Check sheet for the modelled part. Datum: model origin and axes. Units: mm. A direction names the side the tool comes from. Give positions to 0.01 mm unless a question says otherwise; leave off trailing zeros. Loops run counter-clockwise (first coordinate to the right, second up) from the corner with the lowest first, then second, coordinate; pieces in that order, holes last. Notation, with made-up numbers: (-10.5, -5) - (-5.5, -5) arc R15 ccw to (-5.5, 9) - close; hole circle Ø6 at (31, 18.5). An arc over 180 degrees is marked (long way). Use one line per item in the form item = value.
from build123d import *

# Parameters (mm, degrees)
BOSS_EXTRUDE1_DEPTH     = 8.5
CUT_EXTRUDE1_DEPTH      = 2
CUT_EXTRUDE1_DEPTH_BACK = 26.602245995
SKETCH2_R               = 2.75
CUT_EXTRUDE2_DEPTH      = 2
CUT_EXTRUDE2_DEPTH_BACK = 0.25
SKETCH2_3_R             = 5
SKETCH2_3_R_2           = 2.75
SKETCH3_R               = 1.75
CUT_EXTRUDE3_DEPTH      = 28.391148205
SKETCH3_3_R             = 3
SKETCH3_3_R_2           = 1.75
CUT_EXTRUDE4_DEPTH      = 5.85
FILLET1_R               = 2
FILLET2_R               = 2
CUT_EXTRUDE5_DEPTH      = 2
SKETCH5_R               = 1.2
BOSS_EXTRUDE2_DEPTH     = 4
FILLET3_R               = 1
FILLET4_R               = 0.5


with BuildPart() as part:
    # Sketch1 → Boss-Extrude1 (new, symmetric)
    with BuildSketch(Plane.XY):
        with BuildLine():
            Line((11.05, 4), (3.970201506, 4))
            ThreePointArc((3.970201506, 4), (-3.590264914, 6.674165907), (2.926174978, 2))
            Line((2.926174978, 2), (22.05, 2))
            Line((22.05, 2), (22.05, -2))
            Line((22.05, -2), (-22.05, -2))
            Line((-22.05, -2), (-22.05, 2))
            Line((-22.05, 2), (-9.85, 2))
            ThreePointArc((-9.85, 2), (-7.870101013, 2.820101013), (-7.05, 4.8))
            ThreePointArc((-7.05, 4.8), (-1.645444408, 11.655290855), (6.281918497, 8))
            Line((6.281918497, 8), (11.05, 8))
            Line((11.05, 8), (11.05, 4))
        make_face()
    extrude(amount=BOSS_EXTRUDE1_DEPTH, both=True)

    # Sketch2 → Cut-Extrude1 (cut, two sides: drawn at the far end of the back side and taken through both)
    with BuildSketch(Plane(origin=(0, 2, 0), x_dir=(1, 0, 0), z_dir=(0, 1, 0)).offset(-CUT_EXTRUDE1_DEPTH_BACK)):
        with Locations(Location((16.3, 0, 0), (0, 0, 180))):
            Circle(SKETCH2_R)
        with Locations(Location((-16.3, 0, 0), (0, 0, 180))):
            Circle(SKETCH2_R)
    extrude(amount=CUT_EXTRUDE1_DEPTH + CUT_EXTRUDE1_DEPTH_BACK, mode=Mode.SUBTRACT)

    # Sketch2<3> → Cut-Extrude2 (cut, two sides: drawn at the far end of the back side and taken through both)
    # profile 1 of 2: a face of its own
    with BuildSketch(Plane(origin=(0, 2, 0), x_dir=(1, 0, 0), z_dir=(0, 1, 0)).offset(-CUT_EXTRUDE2_DEPTH_BACK)):
        with Locations(Location((16.3, 0, 0), (0, 0, 180))):
            Circle(SKETCH2_3_R)
        with Locations(Location((16.3, 0, 0), (0, 0, 180))):
            Circle(SKETCH2_3_R_2, mode=Mode.SUBTRACT)
    # profile 2 of 2: a face of its own
    with BuildSketch(Plane(origin=(0, 2, 0), x_dir=(1, 0, 0), z_dir=(0, 1, 0)).offset(-CUT_EXTRUDE2_DEPTH_BACK)):
        with Locations(Location((-16.3, 0, 0), (0, 0, 180))):
            Circle(SKETCH2_3_R)
        with Locations(Location((-16.3, 0, 0), (0, 0, 180))):
            Circle(SKETCH2_3_R_2, mode=Mode.SUBTRACT)
    extrude(amount=CUT_EXTRUDE2_DEPTH + CUT_EXTRUDE2_DEPTH_BACK, mode=Mode.SUBTRACT)

    # Sketch3 → Cut-Extrude3 (cut, through all)
    with BuildSketch(Plane(origin=(0, 11.85, 0), x_dir=(1, 0, 0), z_dir=(0, 1, 0))):
        with Locations(Location((7.510100753, 0, 0), (0, 0, 225.426920251))):
            Circle(SKETCH3_R)
    extrude(amount=-CUT_EXTRUDE3_DEPTH, mode=Mode.SUBTRACT)

    # Sketch3<3> → Cut-Extrude4 (cut)
    # profile 1 of 2: a face of its own
    with BuildSketch(Plane(origin=(0, 11.85, 0), x_dir=(1, 0, 0), z_dir=(0, 1, 0))):
        with Locations(Location((7.510100753, 0, 0), (0, 0, 245.83322212))):
            Circle(SKETCH3_3_R)
        with Locations(Location((7.510100753, 0, 0), (0, 0, 180))):
            Circle(SKETCH3_3_R_2, mode=Mode.SUBTRACT)
    # profile 2 of 2: a face of its own
    with BuildSketch(Plane(origin=(0, 11.85, 0), x_dir=(1, 0, 0), z_dir=(0, 1, 0))):
        with Locations(Location((7.510100753, 0, 0), (0, 0, 180))):
            Circle(SKETCH3_3_R_2)
    extrude(amount=-CUT_EXTRUDE4_DEPTH, mode=Mode.SUBTRACT)

    # Fillet1
    fillet1_edges = [part.edges().sort_by_distance(p)[0] for p in [
        (22.05, 0, 8.5),
        (-22.05, 0, -8.5),
        (-22.05, 0, 8.5),
    ]]
    fillet(fillet1_edges, radius=FILLET1_R)

    # Fillet2
    # the kernel refuses this fillet: 2 mm, written as the material it adds along each edge
    with BuildSketch(Plane(origin=(6.281918497, 8, -0.075436901), x_dir=(1, 0, 0), z_dir=(0, 0, 1))) as fillet2_piece_1_section:
        with BuildLine():
            CenterArc((1.125003941, 2), FILLET2_R, 215.07061915, 54.92938085)
            ThreePointArc((-0.511884995, 0.850828729), (-0.240944724, 0.434437491), (0, 0))
            Line((0, 0), (1.125003941, 0))
        make_face()
    fillet2_piece_1 = extrude(amount=8.575436901, mode=Mode.PRIVATE)
    fillet2_piece_1 = fillet2_piece_1 - Plane(origin=(7.510100753, 8.184515376, 0), x_dir=(-0.4093940854484991, 0, 0.9123576507049125), z_dir=(0, 1, 0)) * Cylinder(3, 22, mode=Mode.PRIVATE)
    add(fillet2_piece_1)
    with BuildSketch(Plane(origin=(6.281918497, 8, -8.5), x_dir=(1, 0, 0), z_dir=(0, 0, 1))) as fillet2_piece_2_section:
        with BuildLine():
            CenterArc((1.125003941, 2), FILLET2_R, 215.07061915, 54.92938085)
            ThreePointArc((-0.511884995, 0.850828729), (-0.240944724, 0.434437491), (0, 0))
            Line((0, 0), (1.125003941, 0))
        make_face()
    fillet2_piece_2 = extrude(amount=8.575436901, mode=Mode.PRIVATE)
    fillet2_piece_2 = fillet2_piece_2 - Plane(origin=(7.510100753, 8.184515325, 0), x_dir=(-0.4093940854484991, 0, 0.9123576507049125), z_dir=(0, 1, 0)) * Cylinder(3, 22, mode=Mode.PRIVATE)
    add(fillet2_piece_2)
    # the kernel refuses this fillet: 2 mm, written as the material it takes off along each edge
    with BuildSketch(Plane(origin=(11.05, 13, -8.5), x_dir=(-1, 0, 0), z_dir=(0, -1, 0))) as fillet2_2_piece_1_section:
        with BuildLine():
            CenterArc((FILLET2_R, -FILLET2_R), FILLET2_R, 90, 90)
            Line((0, -FILLET2_R), (0, 0))
            Line((0, 0), (FILLET2_R, 0))
        make_face()
    fillet2_2_piece_1 = extrude(amount=14, mode=Mode.PRIVATE)
    fillet2_2_piece_1 = split(fillet2_2_piece_1, bisect_by=Plane(origin=(10.603264122, 2, -8.053264122), z_dir=(0, 1, 0)), keep=Keep.TOP, mode=Mode.PRIVATE)
    add(fillet2_2_piece_1, mode=Mode.SUBTRACT)
    with BuildSketch(Plane(origin=(11.05, 13, 8.5), x_dir=(-1, 0, 0), z_dir=(0, -1, 0))) as fillet2_2_piece_2_section:
        with BuildLine():
            CenterArc((FILLET2_R, FILLET2_R), FILLET2_R, 180, 90)
            Line((0, FILLET2_R), (0, 0))
            Line((0, 0), (FILLET2_R, 0))
        make_face()
    fillet2_2_piece_2 = extrude(amount=14, mode=Mode.PRIVATE)
    fillet2_2_piece_2 = split(fillet2_2_piece_2, bisect_by=Plane(origin=(10.603264122, 2, 8.053264122), z_dir=(0, 1, 0)), keep=Keep.TOP, mode=Mode.PRIVATE)
    add(fillet2_2_piece_2, mode=Mode.SUBTRACT)

    # Sketch4 → Cut-Extrude5 (cut)
    with BuildSketch(Plane.XZ.offset(2)):
        Polygon((10.772129774, 0), (9.141115264, 2.825), (5.879086243, 2.825), (4.248071732, 0), (5.879086243, -2.825), (9.141115264, -2.825), align=None)
    extrude(amount=-CUT_EXTRUDE5_DEPTH, mode=Mode.SUBTRACT)

    # Sketch5 → Boss-Extrude2 (add)
    with BuildSketch(Plane(origin=(0, 2, 0), x_dir=(1, 0, 0), z_dir=(0, 1, 0))):
        Polygon((27.05, 14.3), (27.05, 24.5), (7.05, 24.5), (7.05, 14.3), (10.398631561, 8.5), (22.05, 8.5), (22.05, 5.639745962), align=None)
        with Locations(Location((21.8, 16.8, 0), (0, 0, 180))):
            Circle(SKETCH5_R, mode=Mode.SUBTRACT)
        with Locations(Location((12.3, 16.8, 0), (0, 0, 180))):
            Circle(SKETCH5_R, mode=Mode.SUBTRACT)
    extrude(amount=-BOSS_EXTRUDE2_DEPTH)

    # Fillet3
    fillet3_edges = [part.edges().sort_by_distance(p)[0] for p in [
        (10.398631561, 0, -8.5),
        (22.05, 0, -5.639745962),
    ]]
    fillet(fillet3_edges, radius=FILLET3_R)

    # Fillet4
    fillet4_edges = [part.edges().sort_by_distance(p)[0] for p in [
        (27.05, 0, -24.5),
        (7.05, 0, -24.5),
        (7.05, 0, -14.3),
        (27.05, 0, -14.3),
    ]]
    fillet(fillet4_edges, radius=FILLET4_R)


solid = part.part
Item 1: Mould release check, pull along X, two halves, no side actions. Record for faces 6 (the face through (10.45, 6.03, -7.93)), 7 (the face through (15, 2, -8)), 8 (the face through (7, 6, 2)), 9 (the face through (4.722, 7.67, 1.107)): released by +X, released by -X, zero draft, split by the parting line, or undercut.
Answer block:
face_6 = released by +X
face_7 = zero draft
face_8 = undercut
face_9 = undercut
Item 2: Section check C-C on y = 6.5. Record the boundary of the cut face in (x, z), then the cut area to 3 significant figures.
Answer block:
outline = (-6.84, -8.5) - (-3.68, -8.5) - (-3.68, 8.5) - (-6.84, 8.5) - close; (3.68, -8.5) - (9.05, -8.5) arc R2 ccw to (11.05, -6.5) - (11.05, 6.5) arc R2 ccw to (9.05, 8.5) - (3.68, 8.5) - close; hole circle Ø6 at (7.51, 0)
area = 149 mm2
Item 3: Section check A-A on x = 16.3. Record the boundary of the cut face in (y, z), then the cut area to 3 significant figures.
Answer block:
outline = (-2, -24.5) - (2, -24.5) - (2, -5) - (1.75, -5) - (1.75, -2.75) - (-2, -2.75) - close; (-2, 2.75) - (1.75, 2.75) - (1.75, 5) - (2, 5) - (2, 8.5) - (-2, 8.5) - close
area = 109 mm2
Item 4: Section check B-B on z = -16.8. Record the boundary of the cut face in (x, y).
Answer block:
outline = (7.05, -2) - (11.1, -2) - (11.1, 2) - (7.05, 2) - close; (13.5, -2) - (20.6, -2) - (20.6, 2) - (13.5, 2) - close; (23, -2) - (27.05, -2) - (27.05, 2) - (23, 2) - close
Item 5: Thickness scan on L1, parallel to Z at x = -16.3, y = -1.1; L2, parallel to Z at x = 16.3, y = -1.05; L3, parallel to Y at x = 11, z = -1.5. Record the ranges inside material, lowest first.
Answer block:
L1 = -8.5 to -2.75, 2.75 to 8.5
L2 = -24.5 to -2.75, 2.75 to 8.5
L3 = -2 to 2, 4 to 8
Item 6: Access from +Z, -Z, +X, -X, +Y, -Y to the whole of each face (thin tool, end or side, straight path). Record for faces 1 (the face through (5.898, 5.014, 0.681)), 2 (the face through (8.31, 0.03, -12.12)), 3 (the face through (11.05, 6, 0)), 4 (the face through (9.945, -1.014, -1.432)), 5 (the face through (8, 4, -2)).
Answer block:
face_1 = +Y, -Y
face_2 = -X, +Y, -Y
face_3 = +Z, -Z, +X, +Y
face_4 = -Y
face_5 = +Z, -Z, +X
Item 7: Section check D-D on x = -16.3. Record the boundary of the cut face in (y, z), then the cut area to 3 significant figures.
Answer block:
outline = (-2, -8.5) - (2, -8.5) - (2, -5) - (1.75, -5) - (1.75, -2.75) - (-2, -2.75) - close; (-2, 2.75) - (1.75, 2.75) - (1.75, 5) - (2, 5) - (2, 8.5) - (-2, 8.5) - close
area = 44.9 mm2
Item 8: Gauge pin test, flat ends, axial feed: P1, Ø6, axis at y = 4, z = -2, coming from the +X side; P2, Ø19.5, axis at x = 11, z = -7, coming from the +Y side; P3, Ø4, axis at x = -8.5, y = 6.5, coming from the -Z side. Record the tip position at first contact, or that the pin passes through.
Answer block:
P1 = 22.05
P2 = 11.74
P3 = -8.5
